```python
from build123d import *

# Parameters (mm, degrees)
SKETCH1_W                            = 140.716
SKETCH1_H                            = 139.7
MAIN_BODY_DEPTH                      = 3.175
SKETCH2_R                            = 25.4
SKETCH2_R_2                          = 1.524
SKETCH2_R_3                          = 0.508
CUTS_FOR_EYES_AND_MOTORS_DEPTH       = 4.175
SKETCH3_W                            = 3.2258
SKETCH3_H                            = 6.604
CUT_FOR_ASSEMBLY_SLOTS_DEPTH         = 4.175
SKETCH4_W                            = 3.2258
SKETCH4_H                            = 73.66
SKETCH4_H_2                          = 6.5278
CUT_FOR_NOSE_DEPTH                   = 4.175
SKETCH9_W                            = 3.2258
SKETCH9_H                            = 6.604
SLOT_FOR_MANDIBLE_DEPTH              = 4.175
CUT_FOR_ROUNDED_FACE_FEATURES_DEPTH  = 4.175
SKETCH12_R                           = 1.524
HOLES_FOR_SPACERS_DEPTH              = 4.175
SKETCH13_R                           = 1.5875
CUT_FOR_FACE_PLATE_MOUNT_SCREW_DEPTH = 4.175
SKETCH15_W                           = 37.279626203
SKETCH15_H                           = 16.998263706
EXTENSION_FOR_LIP_MOTOR_DEPTH        = 3.175
SKETCH16_R                           = 0.508
CUT_FOR_LIP_MOTOR_DEPTH              = 4.175
SKETCH18_R                           = 1.5875
CUT_FOR_BRACKET_SCREW_DEPTH          = 4.175
SKETCH19_W                           = 3.2512
SKETCH19_H                           = 6.604
CUT_FOR_GEAR_TAB_DEPTH               = 4.175


with BuildPart() as part:
    # Sketch1 → main body (new body)
    with BuildSketch(Plane.XY):
        with Locations((0, -69.85)):
            Rectangle(SKETCH1_W, SKETCH1_H)
    extrude(amount=MAIN_BODY_DEPTH)

    # Sketch2 → cuts for eyes and motors (cut, through all)
    with BuildSketch(Plane.XY.offset(3.175)):
        with Locations((-33.528, -48.26)):
            Circle(SKETCH2_R)
        with Locations((-6.1468, -65.024)):
            Circle(SKETCH2_R_2)
        with Locations((-60.9092, -65.024)):
            Circle(SKETCH2_R_2)
        with Locations((-36.575996282, -13.412523563)):
            Circle(SKETCH2_R_3)
        with Locations((-8.636008311, -13.438449703)):
            Circle(SKETCH2_R_3)
        Polygon((-11.170114913, -7.086095515), (-34.030105071, -7.064883219), (-34.033051223, -10.239881852), (-35.430050622, -10.238585545), (-35.435942926, -16.588582811), (-34.038943528, -16.589879118), (-34.04188968, -19.764877751), (-11.181899522, -19.786090048), align=None)
    cuts_for_eyes_and_motors = extrude(amount=-CUTS_FOR_EYES_AND_MOTORS_DEPTH, mode=Mode.SUBTRACT)

    # Sketch3 → cut for assembly slots (cut, through all)
    with BuildSketch(Plane.XY.offset(3.175)):
        with Locations((-65.5701, -63.627)):
            Rectangle(SKETCH3_W, SKETCH3_H)
        with Locations((-65.5701, -25.4)):
            Rectangle(SKETCH3_W, SKETCH3_H)
    cut_for_assembly_slots = extrude(amount=-CUT_FOR_ASSEMBLY_SLOTS_DEPTH, mode=Mode.SUBTRACT)

    # Sketch4 → cut for nose (cut, through all)
    with BuildSketch(Plane.XY.offset(3.175)):
        with Locations((0, -71.12)):
            Rectangle(SKETCH4_W, SKETCH4_H)
        with Locations((0, -25.1079)):
            Rectangle(SKETCH4_W, SKETCH4_H_2)
    extrude(amount=-CUT_FOR_NOSE_DEPTH, mode=Mode.SUBTRACT)

    # Sketch9 → slot for mandible (cut, through all)
    with BuildSketch(Plane.XY.offset(3.175)):
        with Locations((-33.3629, -98.044)):
            Rectangle(SKETCH9_W, SKETCH9_H)
        with Locations((-33.3629, -123.698)):
            Rectangle(SKETCH9_W, SKETCH9_H)
    slot_for_mandible = extrude(amount=-SLOT_FOR_MANDIBLE_DEPTH, mode=Mode.SUBTRACT)

    # mirror of assembly slots: cut for assembly slots across plane
    add(cut_for_assembly_slots.mirror(Plane(origin=(0, 0, 0), x_dir=(0, 0, 1), z_dir=(1, 0, 0))), mode=Mode.SUBTRACT)

    # Mirror1: cuts for eyes and motors across plane
    add(cuts_for_eyes_and_motors.mirror(Plane(origin=(0, 0, 0), x_dir=(0, 0, 1), z_dir=(1, 0, 0))), mode=Mode.SUBTRACT)

    # Sketch11 → cut for rounded face features (cut, through all)
    with BuildSketch(Plane.XY.offset(3.175)):
        with BuildLine():
            Line((-70.358, -139.7), (-70.358, -86.36))
            ThreePointArc((-70.358, -86.36), (-55.943359781, -111.56490753), (-48.768, -139.7))
            Line((-48.768, -139.7), (-70.358, -139.7))
        make_face()
        with BuildLine():
            Line((-70.358, 0), (-70.358, -13.97))
            ThreePointArc((-70.358, -13.97), (-64.724440046, -5.321180316), (-55.88, 0))
            Line((-55.88, 0), (-70.358, 0))
        make_face()
    cut_for_rounded_face_features = extrude(amount=-CUT_FOR_ROUNDED_FACE_FEATURES_DEPTH, mode=Mode.SUBTRACT)

    # Mirror2: cut for rounded face features across plane
    add(cut_for_rounded_face_features.mirror(Plane(origin=(0, 0, 0), x_dir=(0, 0, 1), z_dir=(1, 0, 0))), mode=Mode.SUBTRACT)

    # Sketch12 → holes for spacers (cut, through all)
    with BuildSketch(Plane.XY.offset(3.175)):
        with Locations((-57.658, -7.62)):
            Circle(SKETCH12_R)
        with Locations((-60.198, -83.82)):
            Circle(SKETCH12_R)
        with Locations((-50.038, -114.3)):
            Circle(SKETCH12_R)
    holes_for_spacers = extrude(amount=-HOLES_FOR_SPACERS_DEPTH, mode=Mode.SUBTRACT)

    # Mirror3: holes for spacers across plane
    add(holes_for_spacers.mirror(Plane(origin=(0, 0, 0), x_dir=(0, 0, 1), z_dir=(1, 0, 0))), mode=Mode.SUBTRACT)

    # Mirror4: slot for mandible across plane
    add(slot_for_mandible.mirror(Plane(origin=(0, 0, 0), x_dir=(0, 0, 1), z_dir=(1, 0, 0))), mode=Mode.SUBTRACT)

    # Sketch13 → cut for face plate mount screw (cut, through all)
    with BuildSketch(Plane.XY.offset(3.175)):
        with Locations((58.7502, -24.13)):
            Circle(SKETCH13_R)
        with Locations((58.7502, -76.2)):
            Circle(SKETCH13_R)
    cut_for_face_plate_mount_screw = extrude(amount=-CUT_FOR_FACE_PLATE_MOUNT_SCREW_DEPTH, mode=Mode.SUBTRACT)

    # Mirror5: cut for face plate mount screw across plane
    add(cut_for_face_plate_mount_screw.mirror(Plane(origin=(0, 0, 0), x_dir=(0, 0, 1), z_dir=(1, 0, 0))), mode=Mode.SUBTRACT)

    # Sketch15 → extension for lip motor (add)
    with BuildSketch(Plane.XY.offset(3.175)):
        with Locations((-18.639813101, -148.199131853)):
            Rectangle(SKETCH15_W, SKETCH15_H)
    extension_for_lip_motor = extrude(amount=-EXTENSION_FOR_LIP_MOTOR_DEPTH)

    # mirror of extension for lip motor: extension for lip motor across plane
    add(extension_for_lip_motor.mirror(Plane(origin=(0, 0, 0), x_dir=(0, 0, 1), z_dir=(1, 0, 0))))

    # Sketch16 → cut for lip motor (cut, through all)
    with BuildSketch(Plane.XY.offset(3.175)):
        with Locations((-23.622, -149.86)):
            Circle(SKETCH16_R)
        with Locations((-23.622, -121.92)):
            Circle(SKETCH16_R)
        Polygon((-17.272, -124.46), (-29.972, -124.46), (-29.972, -147.32), (-26.797, -147.32), (-26.797, -148.717), (-20.447, -148.717), (-20.447, -147.32), (-17.272, -147.32), align=None)
    cut_for_lip_motor = extrude(amount=-CUT_FOR_LIP_MOTOR_DEPTH, mode=Mode.SUBTRACT)

    # mirror of lip motor: cut for lip motor across plane
    add(cut_for_lip_motor.mirror(Plane(origin=(0, 0, 0), x_dir=(0, 0, 1), z_dir=(1, 0, 0))), mode=Mode.SUBTRACT)

    # Sketch18 → cut for bracket screw (cut, through all)
    with BuildSketch(Plane.XY.offset(3.175)):
        with Locations((-40.0558, -105.41)):
            Circle(SKETCH18_R)
    cut_for_bracket_screw = extrude(amount=-CUT_FOR_BRACKET_SCREW_DEPTH, mode=Mode.SUBTRACT)

    # mirror of bracket screw: cut for bracket screw across plane
    add(cut_for_bracket_screw.mirror(Plane(origin=(0, 0, 0), x_dir=(0, 0, 1), z_dir=(1, 0, 0))), mode=Mode.SUBTRACT)

    # Sketch19 → cut for gear tab (cut, through all)
    with BuildSketch(Plane.XY.offset(3.175)):
        with Locations((-46.050399644, -92.742342074)):
            Rectangle(SKETCH19_W, SKETCH19_H)
    extrude(amount=-CUT_FOR_GEAR_TAB_DEPTH, mode=Mode.SUBTRACT)


solid = part.part
```
Part model, mm, in its own coordinate system. Round coordinates to 2 decimals unless told otherwise and drop trailing zeros. Order: outer loops, then holes, each group sorted by start corner. A loop starts at its lowest first (then second) coordinate and runs counter-clockwise, first axis right, second up. Notation, with made-up numbers: M 47.5,75 L 62.5,75 A12 cw 62.5,93 Z; hole C 37,59 d9. An arc over 180 degrees is marked long. Answer in a Markdown table with one row per item. Add a question column.
Q1. Pin check, flat tips, straight feed: pin 1 (1.6 mm diameter, centred on y = -96.5, z = 2, fed in from -X); pin 2 (1 mm diameter, centred on x = 45.5, z = 2, fed in from -Y); pin 3 (1.5 mm diameter, centred on y = -126, z = 2.5, fed in from -X). Stop position of each tip, or through.
Q2. Wall check: L1, parallel to X at y = -76.2, z = 1.1; L2, parallel to X at y = -48, z = 0.8; L3, parallel to X at y = -147, z = 2.8. Give the ranges that are in metal, low to high. Write a range as from..to.
Q3. Cut at C-C on y = -111. Give the cut face in (x, z) (3 decimals).
Q4. Cut at B-B on z = 1.15. Give the number of separate pieces and of enclosed holes in the cut face, and give its area (3 significant figures).
Q5. Mould opens along Y. For faces 1 (the face through (67.183, -64, 2)), 2 (the face through (-37.28, -148, 2)), 3 (the face through (-59.5, -77.6, 1.6)), 4 (the face through (-43, -139.7, 2)) say: +Y half, -Y half, draft (parallel to the pull), parting line (faces both ways), or undercut.
Q6. Cut at A-A on y = -48.26. Give the cut face in (x, z) (3 decimals), and give its area (3 significant figures).
Established:
| question | item | result |
|---|---|---|
| 1 | pin 1 | stops at x = -63.94 |
| 1 | pin 2 | stops at y = -139.7 |
| 1 | pin 3 | stops at x = -51.44 |
| 2 | L1 | x = -70.36..-60.34, -57.16..-1.61, 1.61..57.16, 60.34..70.36 |
| 2 | L2 | x = -70.36..-58.93, -8.13..-1.61, 1.61..8.13, 58.93..70.36 |
| 2 | L3 | x = -37.28..-29.97, -17.27..17.27, 29.97..37.28 |
| 3 | outline | M -56.174,0 L 56.174,0 L 56.174,3.175 L -56.174,3.175 Z |
| 4 | separate pieces | 1 |
| 4 | enclosed holes | 41 |
| 4 | area | 13,500 mm2 |
| 5 | face 1 | undercut |
| 5 | face 2 | draft |
| 5 | face 3 | undercut |
| 5 | face 4 | -Y half |
| 6 | outline | M -70.358,0 L -58.928,0 L -58.928,3.175 L -70.358,3.175 Z; M -8.128,0 L -1.613,0 L -1.613,3.175 L -8.128,3.175 Z; M 1.613,0 L 8.128,0 L 8.128,3.175 L 1.613,3.175 Z; M 58.928,0 L 70.358,0 L 70.358,3.175 L 58.928,3.175 Z |
| 6 | area | 114 mm2 |
